from build123d import *

# Parameters (mm, degrees)
SKETCH3_R           = 20
BOSS_EXTRUDE1_DEPTH = 40
BOSS_EXTRUDE2_START = -16
BOSS_EXTRUDE2_DEPTH = 16
BOSS_EXTRUDE3_START = -26
BOSS_EXTRUDE3_DEPTH = 50
BOSS_EXTRUDE4_DEPTH = 20
CUT_EXTRUDE1_START  = 12
CUT_EXTRUDE1_DEPTH  = 12


with BuildPart() as part:
    # Sketch3 → Boss-Extrude1 (new body)
    with BuildSketch(Plane(origin=(0, 0, 0), x_dir=(1, 0, 0), z_dir=(0, 1, 0))):
        Circle(SKETCH3_R)
    extrude(amount=BOSS_EXTRUDE1_DEPTH)

    # Sketch4 → Boss-Extrude2 (add)
    with BuildSketch(Plane(origin=(0, 40, 0), x_dir=(1, 0, 0), z_dir=(0, 1, 0)).offset(BOSS_EXTRUDE2_START)):
        Polygon((25, 10), (45, -40), (-45, -40), (-25, 10), (-17.320508076, 10), (17.320508076, 10), align=None)
    extrude(amount=BOSS_EXTRUDE2_DEPTH)

    # Sketch6 → Boss-Extrude3 (add)
    with BuildSketch(Plane(origin=(0, 24, 0), x_dir=(-1, 0, 0), z_dir=(0, -1, 0)).offset(BOSS_EXTRUDE3_START)):
        Polygon((-41, -30), (41, -30), (45, -40), (-45, -40), align=None)
    extrude(amount=BOSS_EXTRUDE3_DEPTH)

    # Sketch7 → Boss-Extrude4 (add)
    with BuildSketch(Plane(origin=(0, 24, 0), x_dir=(-1, 0, 0), z_dir=(0, -1, 0))):
        with BuildLine():
            Line((-6, -19.078784028), (-6, -30))
            Line((-6, -30), (6, -30))
            Line((6, -30), (6, -19.078784028))
            ThreePointArc((6, -19.078784028), (0, -20), (-6, -19.078784028))
        make_face()
    extrude(amount=BOSS_EXTRUDE4_DEPTH)

    # Sketch7_3 → Cut-Extrude1 (cut)
    with BuildSketch(Plane(origin=(0, 24, 0), x_dir=(-1, 0, 0), z_dir=(0, -1, 0)).offset(CUT_EXTRUDE1_START)):
        with BuildLine():
            ThreePointArc((-18.33030278, 8), (-20, 0), (-18.33030278, -8))
            Line((-18.33030278, -8), (18.33030278, -8))
            ThreePointArc((18.33030278, -8), (20, 0), (18.33030278, 8))
            Line((18.33030278, 8), (-18.33030278, 8))
        make_face()
    extrude(amount=CUT_EXTRUDE1_DEPTH, mode=Mode.SUBTRACT)


solid = part.part
For this review, take the finished solid that the model builds, in its own axes (mm). A direction names the side the tool comes from. Give positions to 0.01 mm unless a question says otherwise; leave off trailing zeros. Loops run counter-clockwise (first coordinate to the right, second up) from the corner with the lowest first, then second, coordinate; pieces in that order, holes last. Notation, with made-up numbers: (17.25, 64.5) -> (56.25, 64.5) arc R28 ccw to (56.25, 100.5) -> close; hole circle Ø10 at (58.25, 70.25). An arc over 180 degrees is marked (long way). One line per question, with ' | ' between items.
1) We need section B-B (y = 5). Write out the cut boundary in (x, z).
Resolved:
outline: (-45, 40) -> (-41, 30) -> (-6, 30) -> (-6, 19.08) arc R20 ccw to (-18.33, 8) -> (18.33, 8) arc R20 ccw to (6, 19.08) -> (6, 30) -> (41, 30) -> (45, 40) -> close; (-18.33, -8) arc R20 ccw to (18.33, -8) -> close
2) For faces 4 (the flat face through (-21, 32, -10)), 5 (the flat face through (-23, 24, 14)), 6 (the flat face through (24, 24, 14)), 7 (the cylindrical face through (-2.6, 15.28, -19.83)), 8 (the flat face through (1, 40, 10)), list the 3-axis set-ups (+Z, -Z, +X, -X, +Y, -Y) from which the entire face can be reached by the end or side of a thin tool; tool diameter is ignored.
Resolved:
face 4: -Z, -X, +Y, -Y | face 5: -X, -Y | face 6: +X, -Y | face 7: -Y | face 8: -Z, +X, -X, +Y
3) The part is to be moulded in two halves that separate along Z. For faces 1 (the flat face through (21, 32, -10)), 2 (the flat face through (0, 6, 8)), 3 (the flat face through (-1, 50, 35)), say which applies: +Z half, -Z half, draft (parallel to the pull), parting line (faces both ways), or undercut.
Resolved:
face 1: -Z half | face 2: undercut | face 3: draft
4) We need section D-D (x = 0). Write out the cut boundary in (y, z), plus the area to 3 significant figures.
Resolved:
outline: (0, -20) -> (40, -20) -> (40, 30) -> (50, 30) -> (50, 40) -> (0, 40) -> (0, 30) -> (4, 30) -> (4, 20) -> (0, 20) -> (0, 8) -> (12, 8) -> (12, -8) -> (0, -8) -> close | area: 2,270 mm2
5) We need section A-A (z = 29). Write out the cut boundary in (x, y).
Resolved:
outline: (-40.6, 24) -> (-6, 24) -> (-6, 4) -> (6, 4) -> (6, 24) -> (40.6, 24) -> (40.6, 40) -> (-40.6, 40) -> close
6) We need section C-C (y = 20). Write out the cut boundary in (x, z).
Resolved:
outline: (-45, 40) -> (-41, 30) -> (-6, 30) -> (-6, 19.08) arc R20 ccw (long way) to (6, 19.08) -> (6, 30) -> (41, 30) -> (45, 40) -> close
7) To check wall thickness, follow probe 1 along Z at (x, y) = (12.5, 9.5); probe 2 along Y at (x, z) = (-15.5, 20.5); probe 3 along Z at (x, y) = (34, 45.5). State the ranges of each line that lie inside material, in increasing order.
Resolved:
probe 1: z = -15.61 to -8, 8 to 15.61, 30 to 40 | probe 2: y = 24 to 40 | probe 3: z = 30 to 40
8) Insertion check: pin 1 Ø8 at (x, z) = (-9, -1.5) entering from -Y; pin 2 Ø8.5 at (x, y) = (-22, 34.5) entering from -Z; pin 3 Ø5 at (x, y) = (-1, 43) entering from -Z. Each pin has a flat end and moves straight along its axis. Give the tip position at first contact, or say it passes through.
Resolved:
pin 1: stops at y = 12 | pin 2: stops at z = -10 | pin 3: stops at z = 30
